```python
from build123d import *

# Parameters (mm, degrees)
F0_R     = 5
F1_DEPTH = 40
F2_W     = 50
F2_H     = 15
F3_DEPTH = 2.5


with BuildPart() as f1:
    # F0 (on Front) → F1 (new body)
    with BuildSketch(Plane.XZ):
        Circle(F0_R)
    extrude(amount=F1_DEPTH)

    # F2 (on Top) → F3 (join, symmetric)
    with BuildSketch(Plane.XY):
        with Locations((0.324281, -47.5)):
            Rectangle(F2_W, F2_H)
    extrude(amount=F3_DEPTH, both=True)


solid = f1.part
```
Verification items for the finished model (mm, model axes). A direction names the side the tool comes from. Give positions to 0.01 mm unless a question says otherwise; leave off trailing zeros. Loops run counter-clockwise (first coordinate to the right, second up) from the corner with the lowest first, then second, coordinate; pieces in that order, holes last.
1. Section check C-C, the plane y = -30.5. Enter the section's corners in (x, z), then the cut area to 3 significant figures.
2. Section check A-A, the plane x = 0. Enter the section's corners in (y, z).
3. Thickness scan on line 1 (Y direction, x = -16, z = 1.25); line 2 (X direction, y = -2.5, z = 2.5); line 3 (Z direction, x = -22, y = -51). Record the ranges inside material, lowest first.
4. Section check B-B, the plane z = -1.5. Enter the section's corners in (x, y).
5. Mould release check, pull along Y, two halves, no side actions. Record for faces 1 (the flat face through (0, -55, 0)), 2 (the cylindrical face through (-1.08, -19.72, -4.88)), 3 (the flat face through (-15, -40, 0)): released by +Y, released by -Y, zero draft, split by the parting line, or undercut.
6. Set-up check for faces 4 (the flat face through (0, -40, -3)), 5 (the flat face through (0, -40, 3)), 6 (the flat face through (0, 0, 0)): record each of +Z, -Z, +X, -X, +Y, -Y from which the full face is reachable in a straight line by a thin tool's end or side.
7. Go/stop test with flat-tipped pins: pin 1 Ø16.5 at (x, y) = (6, -44) entering from -Z; pin 2 Ø12 at (x, y) = (-6.5, -46.5) entering from +Z; pin 3 Ø5.5 at (x, z) = (17, 0) entering from +Y; pin 4 Ø2 at (x, z) = (-2, 4.5) entering from -Y. Record where each tip stops, or that it passes through.
8. Section check D-D, the plane x = 20. Enter the section's corners in (y, z), then the cut area to 3 significant figures.
Geometry says:
1. outline: circle Ø10 at (0, 0)
1. area: 78.5 mm2
2. outline: (-55, -2.5) - (-40, -2.5) - (-40, -5) - (0, -5) - (0, 5) - (-40, 5) - (-40, 2.5) - (-55, 2.5) - close
3. line 1: y = -55 to -40
3. line 2: x = -4.33 to 4.33
3. line 3: z = -2.5 to 2.5
4. outline: (-24.68, -55) - (25.32, -55) - (25.32, -40) - (4.77, -40) - (4.77, 0) - (-4.77, 0) - (-4.77, -40) - (-24.68, -40) - close
5. face 1: released by -Y
5. face 2: zero draft
5. face 3: released by +Y
6. face 4: -Z, +X, -X, -Y
6. face 5: +Z, +X, -X, -Y
6. face 6: +Z, -Z, +X, -X, +Y
7. pin 1: stops at z = -5
7. pin 2: stops at z = 2.5
7. pin 3: stops at y = -40
7. pin 4: stops at y = -40
8. outline: (-55, -2.5) - (-40, -2.5) - (-40, 2.5) - (-55, 2.5) - close
8. area: 75.0 mm2
